from build123d import *

# Parameters (mm, degrees)
F0_W     = 35.56
F0_H     = 35.56
F1_DEPTH = 5.08
F2_W     = 19.812
F2_H     = 4.572
F3_DEPTH = 2.54
F4_W     = 19.812
F4_H     = 4.572
F5_DEPTH = 2.54
F6_W     = 20.32
F6_H     = 5.08
F7_DEPTH = 2.54
F8_W     = 20.32
F8_H     = 5.08
F9_DEPTH = 2.54


with BuildPart() as f1:
    # F0 (on Top) → F1 (new body, symmetric)
    with BuildSketch(Plane.XY):
        Rectangle(F0_W, F0_H)
        with BuildLine():
            Line((0.1598524306, -2.5025173611), (4.9278645833, 12.4850260417))
            Line((4.9278645833, 12.4850260417), (10.31875, 12.4850260417))
            Line((10.31875, 12.4850260417), (1.7583767361, -12.7))
            Line((1.7583767361, -12.7), (-4.0624565972, -12.7))
            Line((-4.0624565972, -12.7), (-12.6062934028, 12.4850260417))
            Line((-12.6062934028, 12.4850260417), (-7.2154079861, 12.4850260417))
            Line((-7.2154079861, 12.4850260417), (-2.4749565972, -2.5025173611))
            add(Edge.make_bspline(
                [(-2.4749565972, -2.5025173611), (-2.08359375, -3.8309461806), (-1.6591579861, -5.5948350694)],
                knots=[0, 0, 0, 1, 1, 1], degree=2))
            add(Edge.make_bspline(
                [(-1.6591579861, -5.5948350694), (-1.2347222222, -7.3587239583), (-1.1355034722, -8.0477430556)],
                knots=[0, 0, 0, 1, 1, 1], degree=2))
            add(Edge.make_bspline(
                [(-1.1355034722, -8.0477430556), (-0.942578125, -6.4657552083), (0.1598524306, -2.5025173611)],
                knots=[0, 0, 0, 1, 1, 1], degree=2))
        make_face(mode=Mode.SUBTRACT)
    extrude(amount=F1_DEPTH, both=True)

    # F2 (on face) → F3 (join)
    with BuildSketch(Plane(origin=(0, 17.78, 0), x_dir=(-1, 0, 0), z_dir=(0, 1, 0))):
        Rectangle(F2_W, F2_H)
    extrude(amount=F3_DEPTH)

    # F4 (on face) → F5 (join)
    with BuildSketch(Plane(origin=(-17.78, 0, 0), x_dir=(0, -1, 0), z_dir=(-1, 0, 0))):
        Rectangle(F4_W, F4_H)
    extrude(amount=F5_DEPTH)

    # F6 (on face) → F7 (cut)
    with BuildSketch(Plane.XZ.offset(17.78)):
        Rectangle(F6_W, F6_H)
    extrude(amount=-F7_DEPTH, mode=Mode.SUBTRACT)

    # F8 (on face) → F9 (cut)
    with BuildSketch(Plane.YZ.offset(17.78)):
        Rectangle(F8_W, F8_H)
    extrude(amount=-F9_DEPTH, mode=Mode.SUBTRACT)


solid = f1.part
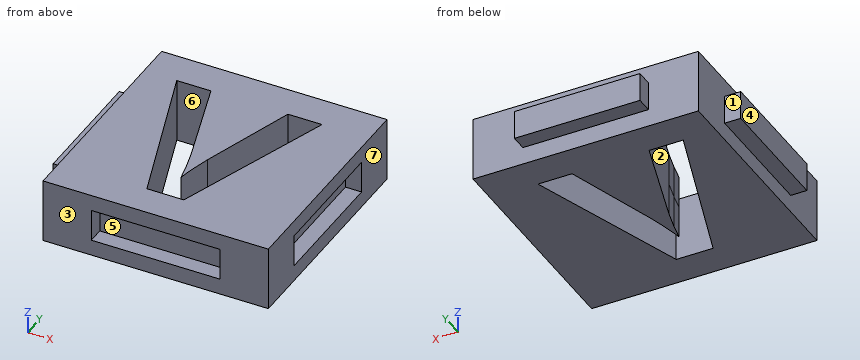
Can you work these out from the model? Positions are in its coordinate system, mm. Face numbers are marked on the shaded views. A direction names the side the tool comes from. Coordinates: 2 decimals unless noted, no trailing zeros. Write each loop counter-clockwise with the first axis right and the second up, starting at its lowest first coordinate (ties: lowest second). Pieces come first, ordered by that corner, then holes. Notation, with made-up numbers: (-4.5, 34) -> (23.5, 34) arc R31 ccw to (23.5, 59) -> close; hole circle Ø2 at (37, -7.75). An arc over 180 degrees is marked (long way). Answer as CSV lines item,"result".
1) If we section it at C-C on x = 13: Please give me the cut outline in (y, z), then the cut area to 3 significant figures.
Check result:
outline,"(-17.78, -5.08) -> (17.78, -5.08) -> (17.78, 5.08) -> (-17.78, 5.08) -> close"
area,"361 mm²"
2) If I drill on line 1 (Y direction, x = 15.5, z = 0.5); line 2 (X direction, y = 11, z = -1.5); line 3 (X direction, y = 1.5, z = -3.5), over which ranges is the centre line in solid material (lowest first)? Write a range as from..to.
Check result:
line 1,"-17.78..-10.16, 10.16..17.78"
line 2,"-17.78..-12.1, -6.75..4.46, 9.81..17.78"
line 3,"-17.78..-8.88, -3.74..1.43, 6.58..17.78"
3) If we section it at A-A on y = -8.5: Please give me the cut outline in (x, z), then the cut area to 3 significant figures.
Check result:
outline,"(-20.32, -2.29) -> (-17.78, -2.29) -> (-17.78, -5.08) -> (-5.49, -5.08) -> (-5.49, 5.08) -> (-17.78, 5.08) -> (-17.78, 2.29) -> (-20.32, 2.29) -> close; (3.19, -5.08) -> (17.78, -5.08) -> (17.78, -2.54) -> (15.24, -2.54) -> (15.24, 2.54) -> (17.78, 2.54) -> (17.78, 5.08) -> (3.19, 5.08) -> close"
area,"272 mm²"
4) If we mould it in two halves opening along Y, with no side actions, what happens to the marked faces 1, 2, 3 and 4? For each: +Y half, -Y half, draft (parallel to the pull), parting line (faces both ways), or undercut.
Check result:
face 1,"+Y half"
face 2,"undercut"
face 3,"-Y half"
face 4,"draft"
5) If we section it at B-B on y = 3: Please give me the cut outline in (x, z).
Check result:
outline,"(-20.32, -2.29) -> (-17.78, -2.29) -> (-17.78, -5.08) -> (-9.39, -5.08) -> (-9.39, 5.08) -> (-17.78, 5.08) -> (-17.78, 2.29) -> (-20.32, 2.29) -> close; (-4.22, -5.08) -> (1.91, -5.08) -> (1.91, 5.08) -> (-4.22, 5.08) -> close; (7.09, -5.08) -> (17.78, -5.08) -> (17.78, -2.54) -> (15.24, -2.54) -> (15.24, 2.54) -> (17.78, 2.54) -> (17.78, 5.08) -> (7.09, 5.08) -> close"
6) On a 3-axis mill with a long thin cutter (end or side, diameter ignored), from which of +Z, -Z, +X, -X, +Y, -Y can I reach the whole of each face in a straight line? I mean the marked faces 5, 6 and 7. Say none if no direction works.
Check result:
face 5,"-Y"
face 6,"+Z, -Z"
face 7,"+Z, -Z, +X, +Y, -Y"
7) Will these pins go through, and if not, where does the flat tip stop? P1, Ø0.8, axis at x = 17, z = 0.5, coming from the +Y side; P2, Ø2.5, axis at x = 4.5, z = 1, coming from the -Y side; P3, Ø3, axis at x = -19.5, z = 1, coming from the +Y side.
Check result:
P1,"y = 17.78"
P2,"y = -15.24"
P3,"y = 9.91"
